Part model, mm, in its own coordinate system. A direction names the side the tool comes from. Give positions to 0.01 mm unless a question says otherwise; leave off trailing zeros. Order: outer loops, then holes, each group sorted by start corner. A loop starts at its lowest first (then second) coordinate and runs counter-clockwise, first axis right, second up.
from build123d import *

# Parameters (mm, degrees)
SKETCH1_W           = 33
SKETCH1_H           = 18.5
SKETCH1_R           = 4
SKETCH1_W_2         = 3
BOSS_EXTRUDE1_DEPTH = 3
SKETCH1_3_W         = 3
SKETCH1_3_H         = 18.5
BOSS_EXTRUDE2_DEPTH = 20
FILLET1_R           = 3
SKETCH2_R           = 2.5
CUT_EXTRUDE1_DEPTH  = 40.680757301


with BuildPart() as part:
    # Sketch1 → Boss-Extrude1 (new body)
    # profile 1 of 2: a face of its own
    with BuildSketch(Plane.XY):
        with Locations((2.5, 0)):
            Rectangle(SKETCH1_W, SKETCH1_H)
        with Locations((-5, 0)):
            Circle(SKETCH1_R, mode=Mode.SUBTRACT)
        with Locations((9, 0)):
            Circle(SKETCH1_R, mode=Mode.SUBTRACT)
    # profile 2 of 2: a face of its own
    with BuildSketch(Plane.XY):
        with Locations((-15.5, 0)):
            Rectangle(SKETCH1_W_2, SKETCH1_H)
    extrude(amount=BOSS_EXTRUDE1_DEPTH)

    # Sketch1_3 → Boss-Extrude2 (add)
    with BuildSketch(Plane.XY):
        with Locations((-15.5, 0)):
            Rectangle(SKETCH1_3_W, SKETCH1_3_H)
    extrude(amount=BOSS_EXTRUDE2_DEPTH)

    # Fillet1
    fillet1_edges = [part.edges().sort_by_distance(p)[0] for p in [
        (-14, 0, 3),
        (-17, 0, 0),
    ]]
    fillet(fillet1_edges, radius=FILLET1_R)

    # Sketch2 → Cut-Extrude1 (cut, through all)
    with BuildSketch(Plane(origin=(-14, 0, 0), x_dir=(0, 0, -1), z_dir=(1, 0, 0))):
        with Locations((-13, 5)):
            Circle(SKETCH2_R)
        with Locations((-13, -5)):
            Circle(SKETCH2_R)
    extrude(amount=-CUT_EXTRUDE1_DEPTH, mode=Mode.SUBTRACT)


solid = part.part
Item 1: Band-saw the part on C-C on x = 9. List the corners of the cut face in (y, z).
Item 2: Drill centre lines: probe 1 along Y at (x, z) = (-15.7, 13); probe 2 along Y at (x, z) = (9, 1.55); probe 3 along X at (y, z) = (7, 10.75). Where is each one in solid material? Low to high.
Item 3: Drop flat-ended pins along their axis: P1, Ø5, axis at x = 8.5, y = -2.5, coming from the +Z side; P2, Ø5, axis at x = -4.5, y = -3.5, coming from the -Z side; P3, Ø10, axis at y = 1.5, z = 15.5, coming from the +X side. Give the stop position or say it passes through.
Item 4: Which spindle directions (+Z, -Z, +X, -X, +Y, -Y) get a long thin tool onto all of the face, cutting with end or side? Do faces 5 (the face through (-14, 0, 13)), 6 (the face through (2, 0, 0)). Say none if no direction does.
Item 5: Band-saw the part on A-A on y = 0. List the corners of the cut face in (x, z), plus the area to 3 significant figures.
Item 6: Pull direction X, two halves, no side cores. Call faces 1 (the face through (-15.5, 5.1, 15.5)), 2 (the face through (-5.867, -3.905, 1.479)), 3 (the face through (5, 0, 1)), 4 (the face through (-16.14, 0.13, 0.9)): released by +X, released by -X, zero draft, split by the parting line, or undercut.
Item 7: Band-saw the part on D-D on y = 5. List the corners of the cut face in (x, z), plus the area to 3 significant figures.
Item 8: Band-saw the part on B-B on z = 13. List the corners of the cut face in (x, y), plus the area to 3 significant figures.
Working result:
1. outline: (-9.25, 0) - (-4, 0) - (-4, 3) - (-9.25, 3) - close; (4, 0) - (9.25, 0) - (9.25, 3) - (4, 3) - close
2. probe 1: y = -9.25 to -7.5, -2.5 to 2.5, 7.5 to 9.25
2. probe 2: y = -9.25 to -4, 4 to 9.25
2. probe 3: x = -17 to -14
3. P1: stops at z = 3
3. P2: stops at z = 0
3. P3: stops at x = -14
4. face 5: +Z, +X, +Y, -Y
4. face 6: -Z, +X, -X, +Y, -Y
5. outline: (-17, 3) arc R3 ccw to (-14, 0) - (-9, 0) - (-9, 3) - (-11, 3) arc R3 cw to (-14, 6) - (-14, 20) - (-17, 20) - close; (-1, 0) - (5, 0) - (5, 3) - (-1, 3) - close; (13, 0) - (19, 0) - (19, 3) - (13, 3) - close
5. area: 111 mm2
6. face 1: zero draft
6. face 2: undercut
6. face 3: undercut
6. face 4: released by -X
7. outline: (-17, 3) arc R3 ccw to (-14, 0) - (19, 0) - (19, 3) - (-11, 3) arc R3 cw to (-14, 6) - (-14, 10.5) - (-17, 10.5) - close; (-17, 15.5) - (-14, 15.5) - (-14, 20) - (-17, 20) - close
7. area: 144 mm2
8. outline: (-17, -9.25) - (-14, -9.25) - (-14, -7.5) - (-17, -7.5) - close; (-17, -2.5) - (-14, -2.5) - (-14, 2.5) - (-17, 2.5) - close; (-17, 7.5) - (-14, 7.5) - (-14, 9.25) - (-17, 9.25) - close
8. area: 25.5 mm2
